from build123d import *

# Parameters (mm, degrees)
F0_W     = 19.05
F0_H     = 50.8
F1_DEPTH = 152.4


with BuildPart() as f1:
    # F0 (on Front) → F1 (new body)
    with BuildSketch(Plane.XZ):
        with Locations((-15.875, 9.525)):
            Rectangle(F0_W, F0_H)
        with BuildLine():
            ThreePointArc((-25.4, -33.3375), (-24.935032, -34.460032), (-23.8125, -34.925))
            Line((-23.8125, -34.925), (25.4, -34.925))
            Line((25.4, -34.925), (25.4, -15.875))
            Line((25.4, -15.875), (-6.35, -15.875))
            Line((-6.35, -15.875), (-25.4, -15.875))
            Line((-25.4, -15.875), (-25.4, -33.3375))
        make_face()
    extrude(amount=F1_DEPTH)


solid = f1.part
Model file for the job. Use its own axes, mm. A direction names the side the tool comes from. Give positions to 0.01 mm unless a question says otherwise; leave off trailing zeros. Loops run counter-clockwise (first coordinate to the right, second up) from the corner with the lowest first, then second, coordinate; pieces in that order, holes last. Notation, with made-up numbers: (72.25, 28.25) -> (114.25, 28.25) arc R17 cw to (114.25, 35.25) -> close; hole circle Ø1 at (-11, 82). An arc over 180 degrees is marked (long way). Use a Markdown table: item, result. Add a question column.
(1) Tool access for faces 1 (the flat face through (-25.4, -75, 1)), 2 (the flat face through (-6.35, -75, 9)): list every direction of +Z, -Z, +X, -X, +Y, -Y with a clear straight run to the whole face (end or side of a thin tool).
(2) Slice it at C-C on z = 22. List the corners of the cut face in (x, y).
(3) Drop flat-ended pins along their axis: pin 1 Ø9.5 at (x, y) = (3.5, -57.5) entering from +Z (3 decimals); pin 2 Ø1 at (y, z) = (-92, 2) entering from +X; pin 3 Ø10 at (x, z) = (3.5, -10) entering from +Y. Give the stop position or say it passes through.
(4) Slice it at B-B on x = 14. List the corners of the cut face in (y, z) (3 decimals).
(5) Wall check: line 1 along X through (y, z) = (-126, 21); line 2 along Z through (x, y) = (9.5, -104.5) (3 decimals). Give the ranges that are in metal, low to high.
Filled sheet:
| question | item | result |
|---|---|---|
| 1 | face 1 | +Z, -Z, -X, +Y, -Y |
| 1 | face 2 | +Z, +X, +Y, -Y |
| 2 | outline | (-25.4, -152.4) -> (-6.35, -152.4) -> (-6.35, 0) -> (-25.4, 0) -> close |
| 3 | pin 1 | z = -15.875 |
| 3 | pin 2 | x = -6.35 |
| 3 | pin 3 | through |
| 4 | outline | (-152.4, -34.925) -> (0, -34.925) -> (0, -15.875) -> (-152.4, -15.875) -> close |
| 5 | line 1 | -25.4 to -6.35 |
| 5 | line 2 | -34.925 to -15.875 |
